```python
from build123d import *

# Parameters (mm, degrees)
F0_W     = 86
F0_H     = 14
F1_DEPTH = 4
F3_DEPTH = 4
F5_DEPTH = 2
F6_R     = 0.25


with BuildPart() as f1:
    # F0 (on Top) → F1 (new body)
    with BuildSketch(Plane.XY):
        Rectangle(F0_W, F0_H)
    extrude(amount=F1_DEPTH)

    # F2 (on face) → F3 (cut)
    with BuildSketch(Plane.XY.offset(4)):
        with BuildLine():
            ThreePointArc((35, -2), (36.4142139414, -1.4142137697), (37.0000005863, 0))
            ThreePointArc((37.0000005863, 0), (36.4142139414, 1.4142137697), (35, 2))
            Line((35, 2), (35, -2))
        make_face()
        with BuildLine():
            Line((35, -2), (35, 2))
            ThreePointArc((35, 2), (33.0000005863, 0), (35, -2))
        make_face()
        with BuildLine():
            ThreePointArc((35, -2), (33.0000005863, 0), (35, 2))
            Line((35, 2), (11, 2))
            ThreePointArc((11, 2), (12.4142135624, 1.4142135624), (13, 0))
            ThreePointArc((13, 0), (12.4142135624, -1.4142135624), (11, -2))
            Line((11, -2), (35, -2))
        make_face()
        with BuildLine():
            Line((11, -2), (11, 2))
            ThreePointArc((11, 2), (9, 0), (11, -2))
        make_face()
        with BuildLine():
            ThreePointArc((13, 0), (12.4142135624, 1.4142135624), (11, 2))
            Line((11, 2), (11, -2))
            ThreePointArc((11, -2), (12.4142135624, -1.4142135624), (13, 0))
        make_face()
    extrude(amount=-F3_DEPTH, mode=Mode.SUBTRACT)

    # F4 (on face) → F5 (cut)
    with BuildSketch(Plane.XY.offset(4)):
        with BuildLine():
            ThreePointArc((35.0000005863, -4), (37.8284277111, -2.8284271247), (39.0000005863, 0))
            ThreePointArc((39.0000005863, 0), (37.8284277111, 2.8284271247), (35.0000005863, 4))
            Line((35.0000005863, 4), (35.0000005863, -4))
        make_face()
        with BuildLine():
            Line((35.0000005863, -4), (35.0000005863, 4))
            ThreePointArc((35.0000005863, 4), (31.0000005863, 0), (35.0000005863, -4))
        make_face()
        with BuildLine():
            ThreePointArc((35.0000005863, -4), (31.0000005863, 0), (35.0000005863, 4))
            Line((35.0000005863, 4), (11.0000005863, 4))
            ThreePointArc((11.0000005863, 4), (13.828427332, 2.8284269175), (15, 0))
            ThreePointArc((15, 0), (13.828427332, -2.8284269175), (11.0000005863, -4))
            Line((11.0000005863, -4), (35.0000005863, -4))
        make_face()
        with BuildLine():
            Line((11.0000005863, -4), (11.0000005863, 4))
            ThreePointArc((11.0000005863, 4), (7, 0), (11.0000005863, -4))
        make_face()
        with BuildLine():
            ThreePointArc((15, 0), (13.828427332, 2.8284269175), (11.0000005863, 4))
            Line((11.0000005863, 4), (11.0000005863, -4))
            ThreePointArc((11.0000005863, -4), (13.828427332, -2.8284269175), (15, 0))
        make_face()
    extrude(amount=-F5_DEPTH, mode=Mode.SUBTRACT)

    # F6
    f6_edges = [f1.edges().sort_by_distance(p)[0] for p in [
        (23.000001, 4, 2),
        (7, 0, 2),
        (23.000001, -4, 2),
        (39.000001, 0, 2),
        (23.000001, -4, 4),
        (7, 0, 4),
        (23.000001, 4, 4),
        (39.000001, 0, 4),
    ]]
    fillet(f6_edges, radius=F6_R)


solid = f1.part
```
Work out the finished part from the listing and answer in its coordinate system (mm). A direction names the side the tool comes from. Coordinates: 2 decimals unless noted, no trailing zeros. Loops run counter-clockwise (first coordinate to the right, second up) from the corner with the lowest first, then second, coordinate; pieces in that order, holes last. Notation, with made-up numbers: (51.25, -8.5) -> (78.25, -8.5) arc R11 ccw to (78.25, 7.5) -> close; hole circle Ø5 at (71, 2). An arc over 180 degrees is marked (long way). Answer as CSV lines item,"result".
Q1. This flat-tipped pin is pushed along its axis until it touches: pin 1 (5 mm diameter, centred on x = -19, y = -0.5, fed in from -Z). Where does it stop, or does it pass through?
Findings:
pin 1,"stops at z = 0"
Q2. The part is cut by section A-A on x = 26.5. Write down the section's boundary in (y, z).
Findings:
outline,"(-7, 0) -> (-2, 0) -> (-2, 2) -> (-3.75, 2) arc R0.25 cw to (-4, 2.25) -> (-4, 3.75) arc R0.25 ccw to (-4.25, 4) -> (-7, 4) -> close; (2, 0) -> (7, 0) -> (7, 4) -> (4.25, 4) arc R0.25 ccw to (4, 3.75) -> (4, 2.25) arc R0.25 cw to (3.75, 2) -> (2, 2) -> close"
Q3. Find the intervals of material crossed by probe 1 along Y at (x, z) = (13, 2.75); probe 2 along Y at (x, z) = (25.5, 0.7); probe 3 along Z at (x, y) = (25, -3), in increasing order.
Findings:
probe 1,"y = -7 to -4, 4 to 7"
probe 2,"y = -7 to -2, 2 to 7"
probe 3,"z = 0 to 2"
Q4. For a pull along Y with two mould halves and no side action, classify faces 4 (the face through (-1, 7, 2)), 5 (the face through (-43, 0, 2)), 6 (the face through (23, 2, 1)) as +Y half, -Y half, draft (parallel to the pull), parting line (faces both ways), or undercut.
Findings:
face 4,"+Y half"
face 5,"draft"
face 6,"undercut"
Q5. A tool of negligible diameter and unlimited length cuts with its end or side. For faces 1 (the face through (9, 0, 1)), 2 (the face through (-1, -7, 2)), 3 (the face through (7, 0, 3)), from which of +Z, -Z, +X, -X, +Y, -Y can it reach the whole face along a straight path? Write none if from no direction.
Findings:
face 1,"+Z, -Z"
face 2,"+Z, -Z, +X, -X, -Y"
face 3,"+Z"
